```python
from build123d import *
from build123d.topology import SkipClean

# Parameters (mm, degrees)
SKETCH1_W           = 120
SKETCH1_H           = 40
SKETCH1_R           = 7.5
SKETCH1_R_2         = 10
BOSS_EXTRUDE1_DEPTH = 20
BOSS_EXTRUDE2_START = 10
SKETCH2_R           = 10
SKETCH2_R_2         = 7.5
BOSS_EXTRUDE2_DEPTH = 10
SKETCH3_W           = 40
SKETCH3_H           = 10
BOSS_EXTRUDE3_DEPTH = 250


with BuildPart() as part:
    # Sketch1 → Boss-Extrude1 (new body)
    with BuildSketch(Plane(origin=(0, 0, 0), x_dir=(1, 0, 0), z_dir=(0, 1, 0))):
        Rectangle(SKETCH1_W, SKETCH1_H)
        with Locations(Location((-40, 0, 0), (0, 0, 270))):
            Circle(SKETCH1_R, mode=Mode.SUBTRACT)
        with Locations(Location((40, 0, 0), (0, 0, 270))):
            Circle(SKETCH1_R_2, mode=Mode.SUBTRACT)
    extrude(amount=BOSS_EXTRUDE1_DEPTH)

    # Sketch2 → Boss-Extrude2 (add)
    with SkipClean():  # the faces are left unmerged after this step: merging them gives an invalid solid
        with BuildSketch(Plane.XZ.offset(BOSS_EXTRUDE2_START)):
            with Locations(Location((-40, 0, 0), (0, 0, 270))):
                Circle(SKETCH2_R)
            with Locations(Location((-40, 0, 0), (0, 0, 270))):
                Circle(SKETCH2_R_2, mode=Mode.SUBTRACT)
        extrude(amount=-BOSS_EXTRUDE2_DEPTH)

    # Sketch3 → Boss-Extrude3 (add)
    with SkipClean():  # the faces are left unmerged after this step: merging them gives an invalid solid
        with BuildSketch(Plane.XY.offset(20)):
            with Locations((40, 15)):
                Rectangle(SKETCH3_W, SKETCH3_H)
        extrude(amount=BOSS_EXTRUDE3_DEPTH)


solid = part.part
```
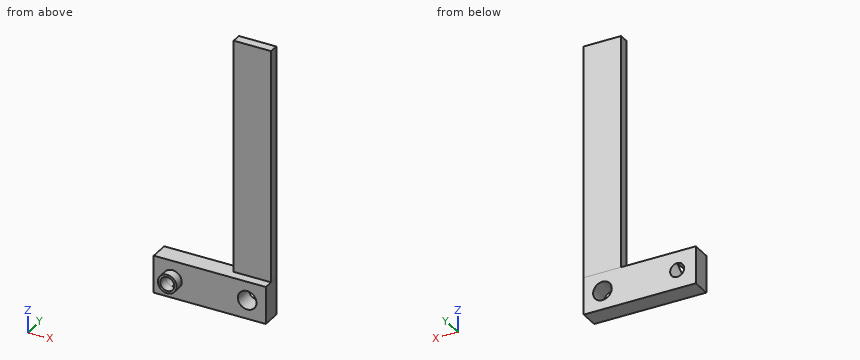
The model under review builds one solid part; all positions refer to its coordinate system, in mm. Round coordinates to 2 decimals unless told otherwise and drop trailing zeros. Order: outer loops, then holes, each group sorted by start corner. A loop starts at its lowest first (then second) coordinate and runs counter-clockwise, first axis right, second up. Notation, with made-up numbers: (47.5, 57.25) -> (87.5, 57.25) arc R6 cw to (87.5, 65.25) -> close; hole circle Ø5 at (42, 18.25). An arc over 180 degrees is marked (long way). Use a Markdown table: item, result.
Q1. We need section D-D on z = 63.5. Write out the cut boundary in (x, y).
Values:
| item | result |
|---|---|
| outline | (20, 10) -> (60, 10) -> (60, 20) -> (20, 20) -> close |
Q2. Clearance check with flat-ended pins moving along their axes: P1, Ø5, axis at x = -34.5, y = 4, coming from the +Z side; P2, Ø12, axis at y = -1, z = 237, coming from the +X side; P3, Ø12, axis at x = 15, z = -3.5, coming from the -Y side; P4, Ø5, axis at y = 17.5, z = 160.5, coming from the -X side. State where each tip first meets the part, or that it passes through.
Values:
| item | result |
|---|---|
| P1 | stops at z = 20 |
| P2 | passes through |
| P3 | stops at y = 0 |
| P4 | stops at x = 20 |
Q3. We need section B-B on x = 40. Write out the cut boundary in (y, z).
Values:
| item | result |
|---|---|
| outline | (0, -20) -> (20, -20) -> (20, -10) -> (0, -10) -> close; (0, 10) -> (20, 10) -> (20, 270) -> (10, 270) -> (10, 20) -> (0, 20) -> close |
